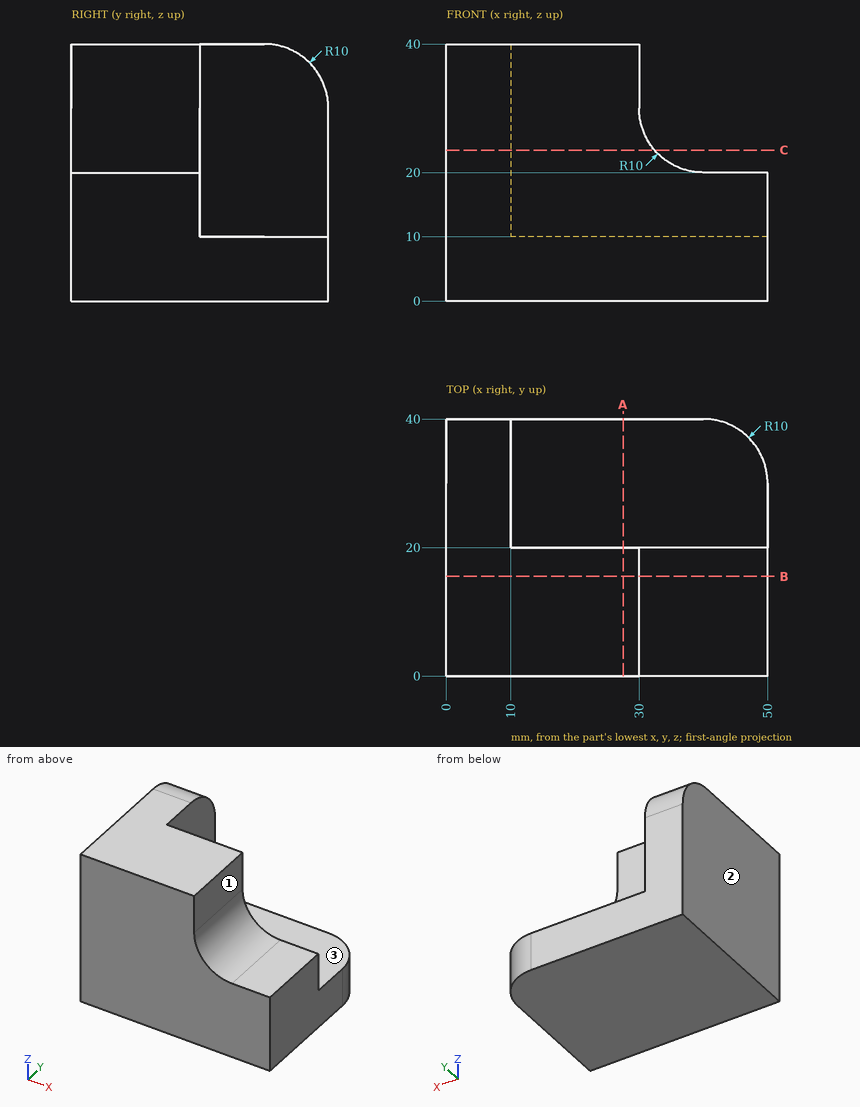
Study the drawing (mm; zero at the part's minimum x, y, z) and answer. A direction names the side the tool comes from. Give positions to 0.01 mm unless a question says otherwise; leave off trailing zeros. Order: outer loops, then holes, each group sorted by start corner. A loop starts at its lowest first (then second) coordinate and runs counter-clockwise, first axis right, second up. Notation, with made-up numbers: M 62,66.25 L 119,66.25 A18 cw 119,84.25 Z; hole C 70,75 d4. An arc over 180 degrees is marked long. Put each result on its own line as item: value. Start each with the question number.
Item 1: Which of the six approach directions +Z, -Z, +X, -X, +Y, -Y give full straight-line access (tool end or side, diameter ignored) to the marked faces 1, 2 and 3?
Item 2: The part is cut by section A-A, the plane x = 27.5. Determine the outline of the cut face in (y, z), and give its area (3 significant figures).
Item 3: Flat-ended cylindrical pins translate along their axes: P1, Ø1.5, axis at x = 44.5, z = 7.5, coming from the +Y side; P2, Ø3, axis at x = 13, z = 28.5, coming from the +Y side; P3, Ø10, axis at x = 21, y = 30.5, coming from the +Z side. Find the tip coordinate at first contact, or state that the pin passes through.
Item 4: Find the intervals of material crossed by line 1 along X through (y, z) = (29, 38.5); line 2 along Y through (x, z) = (25.5, 19.5), in increasing order.
Item 5: The part is cut by section C-C, the plane z = 23.5. Determine the outline of the cut face in (x, y), and give its area (3 significant figures).
Item 6: The part is cut by section B-B, the plane y = 15.5. Determine the outline of the cut face in (x, z), and give its area (3 significant figures).
Answer key:
1. face 1: +Z, +X, +Y, -Y
1. face 2: +Z, -Z, -X, +Y, -Y
1. face 3: +Z, +X, +Y
2. outline: M 0,0 L 40,0 L 40,10 L 20,10 L 20,40 L 0,40 Z
2. area: 1,000 mm²
3. P1: stops at y = 39.27
3. P2: stops at y = 20
3. P3: stops at z = 10
4. line 1: x = 0 to 10
4. line 2: y = 0 to 20
5. outline: M 0,0 L 32.4,0 L 32.4,20 L 10,20 L 10,40 L 0,40 Z
5. area: 848 mm²
6. outline: M 0,0 L 50,0 L 50,20 L 40,20 A10 cw 30,30 L 30,40 L 0,40 Z
6. area: 1,620 mm²
